The model under review builds one solid part; all positions refer to its coordinate system, in mm. Face numbers are marked on the shaded views. A direction names the side the tool comes from. Give positions to 0.01 mm unless a question says otherwise; leave off trailing zeros. Order: outer loops, then holes, each group sorted by start corner. A loop starts at its lowest first (then second) coordinate and runs counter-clockwise, first axis right, second up. Notation, with made-up numbers: (28, 73.5) - (33, 73.5) arc R18 ccw to (33, 80.5) - close; hole circle Ø10 at (-36, 15.25). An arc over 180 degrees is marked (long way). Write item = value, one per line. Start each with the question number.
1. Machinability: for the marked faces 1, 2 and 3, which of the approach directions +Z, -Z, +X, -X, +Y, -Y give a long, thin tool a straight path to every point of the face, cutting with its end or side? Answer none if there is none.
2. We need section B-B, the plane z = 0. Give the boundary of the cut face in (x, y).
3. Mouldability with a two-part tool opening along Z and no side actions: class the marked faces 4, 5 and 6 as pulls with the +Z half, pulls with the -Z half, needs draft (parallel to the pull), parting line crosses it, or undercut.
4. For P1, Ø1.5, axis at x = -2.5, y = -6, coming from the -Z side; P2, Ø1, axis at y = -9, z = -2.5, coming from the +X side; P3, Ø4.5, axis at y = -2.5, z = 0, coming from the +X side (1 decimal); P4, Ø1.5, axis at x = -13.5, y = -4.5, coming from the +Z side, all flat-tipped, find the tip position at first contact; note any pin that passes through.
5. We need section D-D, the plane z = 7.5. Give the boundary of the cut face in (x, y), and give its area (3 significant figures).
6. We need section A-A, the plane y = -2.5. Give the boundary of the cut face in (x, z), and give its area (3 significant figures).
7. We need section C-C, the plane x = -12. Give the boundary of the cut face in (y, z), and give its area (3 significant figures).
8. Wall thickness on probe 1 along Y at (x, z) = (-6.25, 0); probe 2 along Y at (x, z) = (-0.6, 0); probe 3 along Z at (x, y) = (-1.25, -6): over which ranges is each line inside the solid? List them lowest first.
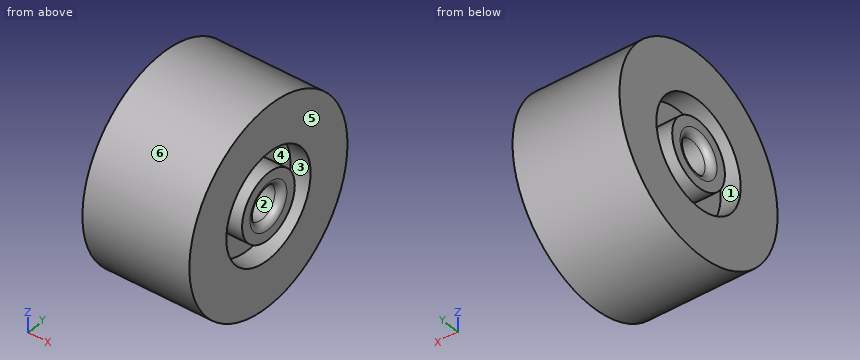
from build123d import *

# Parameters (mm, degrees)
SKETCH2_R          = 2.5
CUT_EXTRUDE1_DEPTH = 16
FILLET1_R          = 1


with BuildPart() as part:
    # Sketch1 → Revolve2 (revolve)
    with BuildSketch(Plane.XY):
        Polygon((0, 2.5), (-3, 2.5), (-3, 5.5), (0, 5.5), (0, 12.5), (-16, 12.5), (-16, 5.5), (-13, 5.5), (-13, 2.5), (-16, 2.5), (-16, -2.5), (0, -2.5), align=None)
    revolve(axis=Axis((8.187259668, -2.5, 0), (-1, 0, 0)))

    # Sketch2 → Cut-Extrude1 (cut)
    with BuildSketch(Plane.ZY.offset(16)):
        with Locations((0, -2.5)):
            Circle(SKETCH2_R)
    extrude(amount=-CUT_EXTRUDE1_DEPTH, mode=Mode.SUBTRACT)

    # Fillet1
    fillet1_edges = [part.edges().sort_by_distance(p)[0] for p in [
        (-16, -2.5, -2.5),
        (0, -2.5, -2.5),
    ]]
    fillet(fillet1_edges, radius=FILLET1_R)


solid = part.part
Model answer:
q1.face_1 = -X
q1.face_2 = +X, -X
q1.face_3 = +X
q2.outline = (-16, -17.5) - (0, -17.5) - (0, -10.5) - (-3, -10.5) - (-3, -7.5) - (0, -7.5) - (0, -6) arc R1 ccw to (-1, -5) - (-15, -5) arc R1 ccw to (-16, -6) - (-16, -7.5) - (-13, -7.5) - (-13, -10.5) - (-16, -10.5) - close; (-16, 1) arc R1 ccw to (-15, 0) - (-1, 0) arc R1 ccw to (0, 1) - (0, 2.5) - (-3, 2.5) - (-3, 5.5) - (0, 5.5) - (0, 12.5) - (-16, 12.5) - (-16, 5.5) - (-13, 5.5) - (-13, 2.5) - (-16, 2.5) - close
q3.face_4 = undercut
q3.face_5 = needs draft
q3.face_6 = parting line crosses it
q4.P1 = -14.75
q4.P2 = -3
q4.P3 = through
q4.P4 = 14.95
q5.outline = (-16, -15.49) - (0, -15.49) - (0, -5.28) - (-3, -5.28) - (-3, 0.28) - (0, 0.28) - (0, 10.49) - (-16, 10.49) - (-16, 0.28) - (-13, 0.28) - (-13, -5.28) - (-16, -5.28) - close
q5.area = 382 mm2
q6.outline = (-16, -15) - (0, -15) - (0, -8) - (-3, -8) - (-3, -5) - (0, -5) - (0, -3.5) arc R1 ccw to (-1, -2.5) - (-15, -2.5) arc R1 ccw to (-16, -3.5) - (-16, -5) - (-13, -5) - (-13, -8) - (-16, -8) - close; (-16, 3.5) arc R1 ccw to (-15, 2.5) - (-1, 2.5) arc R1 ccw to (0, 3.5) - (0, 5) - (-3, 5) - (-3, 8) - (0, 8) - (0, 15) - (-16, 15) - (-16, 8) - (-13, 8) - (-13, 5) - (-16, 5) - close
q6.area = 363 mm2
q7.outline = circle Ø30 at (-2.5, 0); hole circle Ø5 at (-2.5, 0)
q7.area = 687 mm2
q8.probe_1 = -17.5 to -5, 0 to 12.5
q8.probe_2 = -17.5 to -10.5, -7.5 to -5.08, 0.08 to 2.5, 5.5 to 12.5
q8.probe_3 = -14.59 to -7.19, -3.57 to 3.57, 7.19 to 14.59
